Build history of the part. All positions in model axes, mm. A direction names the side the tool comes from. Give positions to 0.01 mm unless a question says otherwise; leave off trailing zeros. Order: outer loops, then holes, each group sorted by start corner. A loop starts at its lowest first (then second) coordinate and runs counter-clockwise, first axis right, second up. Notation, with made-up numbers: (85, -34.75) - (105, -34.75) arc R4 cw to (105, -28.75) - close; hole circle Ø8 at (27.5, -4). An arc over 180 degrees is marked (long way). Use a Markdown table: item, result.
from build123d import *

# Parameters (mm, degrees)
CROQUIS1_R              = 1.5
CROQUIS1_W              = 21.7
CROQUIS1_H              = 10.8
SALIENTE_EXTRUIR1_DEPTH = 3
CORTAR_EXTRUIR2_DEPTH   = 3
REDONDEO1_R             = 1
REDONDEO2_R             = 0.25


with BuildPart() as part:
    # Croquis1 → Saliente-Extruir1 (new body)
    with BuildSketch(Plane.XY):
        with BuildLine():
            Line((-50, 25), (-50, -25))
            ThreePointArc((-50, -25), (-49.267766953, -26.767766953), (-47.5, -27.5))
            Line((-47.5, -27.5), (-37.9, -27.5))
            Line((-37.9, -27.5), (-37.9, -30.5))
            Line((-37.9, -30.5), (-32.9, -30.5))
            Line((-32.9, -30.5), (-32.9, -33.5))
            Line((-32.9, -33.5), (-37.9, -33.5))
            Line((-37.9, -33.5), (-37.9, -36.5))
            Line((-37.9, -36.5), (-30.4, -36.5))
            ThreePointArc((-30.4, -36.5), (-28.632233047, -35.767766953), (-27.9, -34))
            Line((-27.9, -34), (-27.9, -27.5))
            Line((-27.9, -27.5), (27.9, -27.5))
            Line((27.9, -27.5), (27.9, -34))
            ThreePointArc((27.9, -34), (28.632233047, -35.767766953), (30.4, -36.5))
            Line((30.4, -36.5), (37.9, -36.5))
            Line((37.9, -36.5), (37.9, -33.5))
            Line((37.9, -33.5), (32.9, -33.5))
            Line((32.9, -33.5), (32.9, -30.5))
            Line((32.9, -30.5), (37.9, -30.5))
            Line((37.9, -30.5), (37.9, -27.5))
            Line((37.9, -27.5), (47.5, -27.5))
            ThreePointArc((47.5, -27.5), (49.267766953, -26.767766953), (50, -25))
            Line((50, -25), (50, 25))
            ThreePointArc((50, 25), (49.267766953, 26.767766953), (47.5, 27.5))
            Line((47.5, 27.5), (37.9, 27.5))
            Line((37.9, 27.5), (37.9, 30.5))
            Line((37.9, 30.5), (32.9, 30.5))
            Line((32.9, 30.5), (32.9, 33.5))
            Line((32.9, 33.5), (37.9, 33.5))
            Line((37.9, 33.5), (37.9, 36.5))
            Line((37.9, 36.5), (30.4, 36.5))
            ThreePointArc((30.4, 36.5), (28.632233047, 35.767766953), (27.9, 34))
            Line((27.9, 34), (27.9, 27.5))
            Line((27.9, 27.5), (-27.9, 27.5))
            Line((-27.9, 27.5), (-27.9, 34))
            ThreePointArc((-27.9, 34), (-28.632233047, 35.767766953), (-30.4, 36.5))
            Line((-30.4, 36.5), (-37.9, 36.5))
            Line((-37.9, 36.5), (-37.9, 33.5))
            Line((-37.9, 33.5), (-32.9, 33.5))
            Line((-32.9, 33.5), (-32.9, 30.5))
            Line((-32.9, 30.5), (-37.9, 30.5))
            Line((-37.9, 30.5), (-37.9, 27.5))
            Line((-37.9, 27.5), (-47.5, 27.5))
            ThreePointArc((-47.5, 27.5), (-49.267766953, 26.767766953), (-50, 25))
        make_face()
        with Locations((-14, 17.663397979)):
            Circle(CROQUIS1_R, mode=Mode.SUBTRACT)
        with Locations(Location((14, 17.663397979, 0), (0, 0, 180))):
            Circle(CROQUIS1_R, mode=Mode.SUBTRACT)
        with Locations((14, 3.643397979)):
            Circle(CROQUIS1_R, mode=Mode.SUBTRACT)
        with Locations(Location((-14, 3.643397979, 0), (0, 0, 180))):
            Circle(CROQUIS1_R, mode=Mode.SUBTRACT)
        with Locations((0, 10.653397979)):
            Rectangle(CROQUIS1_W, CROQUIS1_H, mode=Mode.SUBTRACT)
    extrude(amount=SALIENTE_EXTRUIR1_DEPTH)

    # Croquis2 → Cortar-Extruir2 (cut, symmetric)
    with BuildSketch(Plane.XY):
        with BuildLine():
            Line((-17.5, -17.5), (17.5, -17.5))
            ThreePointArc((17.5, -17.5), (19.267766953, -18.232233047), (20, -20))
            Line((20, -20), (20, -37.5))
            Line((20, -37.5), (-20, -37.5))
            Line((-20, -37.5), (-20, -20))
            ThreePointArc((-20, -20), (-19.267766953, -18.232233047), (-17.5, -17.5))
        make_face()
    extrude(amount=CORTAR_EXTRUIR2_DEPTH, both=True, mode=Mode.SUBTRACT)

    # Redondeo1
    redondeo1_edges = [part.edges().sort_by_distance(p)[0] for p in [
        (10.85, 5.253397979, 1.5),
        (10.85, 16.053397979, 1.5),
        (-10.85, 16.053397979, 1.5),
        (-10.85, 5.253397979, 1.5),
        (-37.9, -27.5, 1.5),
        (-37.9, 27.5, 1.5),
        (-37.9, 36.5, 1.5),
        (-27.9, 27.5, 1.5),
        (27.9, 27.5, 1.5),
        (37.9, 36.5, 1.5),
        (37.9, 27.5, 1.5),
        (37.9, -27.5, 1.5),
        (37.9, -36.5, 1.5),
        (27.9, -27.5, 1.5),
        (-27.9, -27.5, 1.5),
        (-37.9, -36.5, 1.5),
    ]]
    fillet(redondeo1_edges, radius=REDONDEO1_R)

    # Redondeo2
    redondeo2_edges = [part.edges().sort_by_distance(p)[0] for p in [
        (20, -27.5, 1.5),
        (-20, -27.5, 1.5),
        (-37.9, 30.5, 1.5),
        (-32.9, 30.5, 1.5),
        (-32.9, 33.5, 1.5),
        (-37.9, 33.5, 1.5),
        (37.9, 33.5, 1.5),
        (32.9, 33.5, 1.5),
        (32.9, 30.5, 1.5),
        (37.9, 30.5, 1.5),
        (37.9, -30.5, 1.5),
        (32.9, -30.5, 1.5),
        (32.9, -33.5, 1.5),
        (37.9, -33.5, 1.5),
        (-37.9, -33.5, 1.5),
        (-32.9, -33.5, 1.5),
        (-32.9, -30.5, 1.5),
        (-37.9, -30.5, 1.5),
    ]]
    fillet(redondeo2_edges, radius=REDONDEO2_R)


solid = part.part
1) Two-plate mould, pull along Y, no slides. Class faces 5 (the cylindrical face through (-28.613, 35.748, 1.479)), 6 (the cylindrical face through (-12.894, 2.63, 1.479)), 7 (the flat face through (27.9, 31, 1)): +Y half, -Y half, draft (parallel to the pull), parting line (faces both ways), or undercut.
Computed:
| item | result |
|---|---|
| face 5 | +Y half |
| face 6 | undercut |
| face 7 | draft |
2) Slice it at D-D (x = 42). Write the cut outline in (y, z), and give its area (3 significant figures).
Computed:
| item | result |
|---|---|
| outline | (-27.5, 0) - (27.5, 0) - (27.5, 3) - (-27.5, 3) - close |
| area | 165 mm² |
3) Slice it at C-C (x = 1). Write the cut outline in (y, z).
Computed:
| item | result |
|---|---|
| outline | (-17.5, 0) - (5.25, 0) - (5.25, 3) - (-17.5, 3) - close; (16.05, 0) - (27.5, 0) - (27.5, 3) - (16.05, 3) - close |
4) Pin check, flat tips, straight feed: P1, Ø1, axis at x = 0, z = 1, coming from the -Y side; P2, Ø0.9, axis at y = 34.5, z = 1, coming from the -X side; P3, Ø1.4, axis at y = 34.5, z = 1, coming from the +X side. Stop position of each tip, or through.
Computed:
| item | result |
|---|---|
| P1 | stops at y = -17.5 |
| P2 | stops at x = -37.9 |
| P3 | stops at x = 37.9 |
5) Wall check: line 1 (Y direction, x = -14, z = 1.7); line 2 (Y direction, x = 35, z = 2.3); line 3 (X direction, y = 9, z = 1.9). Give the ranges that are in metal, low to high. Write a range as from..to.
Computed:
| item | result |
|---|---|
| line 1 | y = -17.5..2.14, 5.14..16.16, 19.16..27.5 |
| line 2 | y = -36.5..-33.5, -30.5..30.5, 33.5..36.5 |
| line 3 | x = -50..-10.85, 10.85..50 |
6) Slice it at A-A (y = 8.5). Write the cut outline in (x, z), and give its area (3 significant figures).
Computed:
| item | result |
|---|---|
| outline | (-50, 0) - (-10.85, 0) - (-10.85, 3) - (-50, 3) - close; (10.85, 0) - (50, 0) - (50, 3) - (10.85, 3) - close |
| area | 235 mm² |
7) Slice it at B-B (x = 14). Write the cut outline in (y, z), and give its area (3 significant figures).
Computed:
| item | result |
|---|---|
| outline | (-17.5, 0) - (2.14, 0) - (2.14, 3) - (-17.5, 3) - close; (5.14, 0) - (16.16, 0) - (16.16, 3) - (5.14, 3) - close; (19.16, 0) - (27.5, 0) - (27.5, 3) - (19.16, 3) - close |
| area | 117 mm² |
8) Tool access for faces 1 (the flat face through (32.9, 32, 1)), 2 (the flat face through (-27.9, -31, 1)), 3 (the flat face through (-10.85, 11, 1)), 4 (the flat face through (-32.9, 32, 1)): list every direction of +Z, -Z, +X, -X, +Y, -Y with a clear straight run to the whole face (end or side of a thin tool).
Computed:
| item | result |
|---|---|
| face 1 | +Z, -Z, +X |
| face 2 | +Z, -Z, -Y |
| face 3 | +Z, -Z |
| face 4 | +Z, -Z, -X |
